Can you work these out from the model? Positions are in its coordinate system, mm. Face numbers are marked on the shaded views. A direction names the side the tool comes from. Give positions to 0.01 mm unless a question says otherwise; leave off trailing zeros. Write each loop counter-clockwise with the first axis right and the second up, starting at its lowest first coordinate (ties: lowest second). Pieces come first, ordered by that corner, then holes. Notation, with made-up numbers: M 33,27.25 L 57,27.25 A27 ccw 57,51.25 Z; hole C 70.25,47 d8. An arc over 180 degrees is marked long. Use CSV: the item, a comma, the result in double quotes. Start each with the question number.
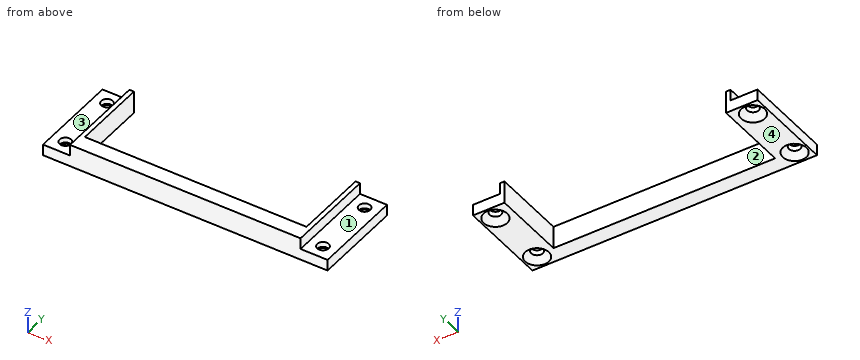
from build123d import *

# Parameters (mm, degrees)
BOSS_EXTRU_1_DEPTH                                = 10
BOSS_EXTRU_1_DEPTH_BACK                           = 0.0001
ESQUISSE1_W                                       = 102.6
ESQUISSE1_H                                       = 35
ESQUISSE4_W                                       = 98.6
ESQUISSE4_H                                       = 51.6
ENL_V_MAT_EXTRU_2_DEPTH                           = 33
ESQUISSE19_W                                      = 102.6
ESQUISSE19_H                                      = 10.0001
BOSS_EXTRU_4_DEPTH                                = 5
ESQUISSE21_W                                      = 5
ESQUISSE21_H                                      = 40
BOSS_EXTRU_5_DEPTH                                = 12
ESQUISSE22_W                                      = 5
ESQUISSE22_H                                      = 40
BOSS_EXTRU_6_DEPTH                                = 12
FRAISAGE_POUR_VIS_T_TE_FRAIS_E_BOMB_E_D           = 5.09999996
FRAISAGE_POUR_VIS_T_TE_FRAIS_E_BOMB_E_CSINK_D     = 10.500000082
FRAISAGE_POUR_VIS_T_TE_FRAIS_E_BOMB_E_CSINK_ANGLE = 90


with BuildPart() as part:
    # Esquisse1 → Boss.-Extru.1 (new, two sides: drawn at the far end of the back side and taken through both)
    with BuildSketch(Plane.XY.offset(-BOSS_EXTRU_1_DEPTH_BACK)):
        with Locations((33.832170394, 1.686746988)):
            Rectangle(ESQUISSE1_W, ESQUISSE1_H)
    extrude(amount=BOSS_EXTRU_1_DEPTH + BOSS_EXTRU_1_DEPTH_BACK)

    # Esquisse4 → Enlèv. mat.-Extru.2 (cut)
    with BuildSketch(Plane(origin=(0, 19.186746988, 0), x_dir=(1, 0, 0), z_dir=(0, 1, 0))):
        with Locations((33.832170394, -25.7999)):
            Rectangle(ESQUISSE4_W, ESQUISSE4_H)
    extrude(amount=-ENL_V_MAT_EXTRU_2_DEPTH, mode=Mode.SUBTRACT)

    # Esquisse19 → Boss.-Extru.4 (add)
    with BuildSketch(Plane.XZ.offset(15.813253012)):
        with Locations((33.832170394, 4.99995)):
            Rectangle(ESQUISSE19_W, ESQUISSE19_H)
    extrude(amount=BOSS_EXTRU_4_DEPTH)

    # Esquisse21 → Boss.-Extru.5 (add)
    with BuildSketch(Plane.ZY.offset(17.467829606)):
        with Locations((2.4999, -0.813253012)):
            Rectangle(ESQUISSE21_W, ESQUISSE21_H)
    extrude(amount=BOSS_EXTRU_5_DEPTH)

    # Esquisse22 → Boss.-Extru.6 (add)
    with BuildSketch(Plane(origin=(85.132170394, 0, 0), x_dir=(0, 0, -1), z_dir=(1, 0, 0))):
        with Locations((-2.4999, -0.813253012)):
            Rectangle(ESQUISSE22_W, ESQUISSE22_H)
    extrude(amount=BOSS_EXTRU_6_DEPTH)

    # Fraisage pour vis à tête fraisée bombée #51 (through all)
    with Locations(Plane(origin=(91.132170394, 13.186746988, -0.0001), x_dir=(-1, 0, 0), z_dir=(0, 0, -1))):
        with Locations((0, 0), (0, -28), (114.6, 0), (114.6, -28)):
            CounterSinkHole(FRAISAGE_POUR_VIS_T_TE_FRAIS_E_BOMB_E_D / 2, FRAISAGE_POUR_VIS_T_TE_FRAIS_E_BOMB_E_CSINK_D / 2, counter_sink_angle=FRAISAGE_POUR_VIS_T_TE_FRAIS_E_BOMB_E_CSINK_ANGLE)


solid = part.part
(1) I want a section at C-C (z = 8.25). Write out the boundary of the cut face in (x, y), and give its area (3 significant figures).
(2) Will these pins go through, and if not, where does the flat tip stop? pin 1 Ø6.5 at (x, y) = (91.13, -14.81) entering from -Z; pin 2 Ø3 at (x, z) = (11.5, 3) entering from +Y; pin 3 Ø4.5 at (x, y) = (-23.47, 13.19) entering from -Z; pin 4 Ø9.5 at (x, y) = (92, -5.5) entering from +Z.
(3) I want a section at B-B (z = 1.25). Write out the boundary of the cut face in (x, y), and give its area (3 significant figures).
(4) Please list where these lines run through material, in increasing order: L1, parallel to X at y = 6.5, z = 3.75; L2, parallel to X at y = -7.5, z = 9; L3, parallel to Y at x = 21.5, z = 2.75. Write a range as [from, to].
(5) Thinking about a two-plate mould opening in X: for the marked faces 1 and 2, which applies, released by +X, released by -X, zero draft, split by the parting line, or undercut?
(6) I want a section at D-D (x = 54). Write out the boundary of the cut face in (y, z).
(7) I want a section at A-A (y = 6). Write out the boundary of the cut face in (x, z).
(8) Which directions (+Z, -Z, +X, -X, +Y, -Y) give clear straight access to the entire face, cutting with the end or side of a thin tool? Please do the marked faces 3 and 4.
Geometry results:
1,outline,"M -17.47,-20.81 L 85.13,-20.81 L 85.13,19.19 L 83.13,19.19 L 83.13,-13.81 L -15.47,-13.81 L -15.47,19.19 L -17.47,19.19 Z"
1,area,"850 mm2"
2,pin 1,"stops at z = 2"
2,pin 2,"stops at y = -13.81"
2,pin 3,"passes through"
2,pin 4,"stops at z = 5"
3,outline,"M -29.47,-20.81 L 97.13,-20.81 L 97.13,19.19 L 83.13,19.19 L 83.13,-13.81 L -15.47,-13.81 L -15.47,19.19 L -29.47,19.19 Z; hole C -23.47,-14.81 d8; hole C -23.47,13.19 d8; hole C 91.13,-14.81 d8; hole C 91.13,13.19 d8"
3,area,"1,610 mm2"
4,L1,"x = [-29.47, -15.47], [83.13, 97.13]"
4,L2,"x = [-17.47, -15.47], [83.13, 85.13]"
4,L3,"y = [-20.81, -13.81]"
5,face 1,"zero draft"
5,face 2,"undercut"
6,outline,"M -20.81,0 L -13.81,0 L -13.81,10 L -20.81,10 Z"
7,outline,"M -29.47,0 L -15.47,0 L -15.47,10 L -17.47,10 L -17.47,5 L -29.47,5 Z; M 83.13,0 L 97.13,0 L 97.13,5 L 85.13,5 L 85.13,10 L 83.13,10 Z"
8,face 3,"+Z, -X, +Y, -Y"
8,face 4,"-Z, +X, -X, +Y, -Y"
